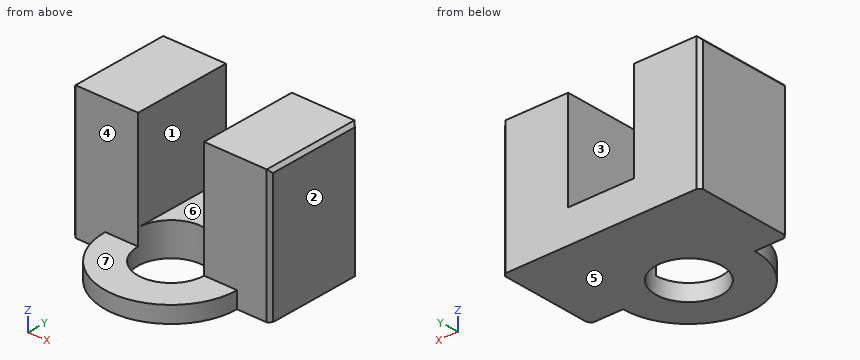
from build123d import *

# Parameters (mm, degrees)
BOSS_EXTRUDE1_DEPTH = 30
SKETCH2_R           = 20
BOSS_EXTRUDE2_DEPTH = 5
SKETCH3_R           = 10
CUT_EXTRUDE1_DEPTH  = 20
CHAMFER1_SIZE       = 1


with BuildPart() as part:
    # Sketch1 → Boss-Extrude1 (new body)
    with BuildSketch(Plane(origin=(0, 0, 0), x_dir=(1, 0, 0), z_dir=(0, 1, 0))):
        Polygon((-30, 0), (-30, -40), (-10, -40), (-10, -10), (10, -10), (10, -40), (30, -40), (30, 0), align=None)
    extrude(amount=BOSS_EXTRUDE1_DEPTH)

    # Sketch2 → Boss-Extrude2 (add)
    with BuildSketch(Plane.XY):
        Circle(SKETCH2_R)
    extrude(amount=BOSS_EXTRUDE2_DEPTH)

    # Sketch3 → Cut-Extrude1 (cut)
    with BuildSketch(Plane.XY):
        Circle(SKETCH3_R)
    extrude(amount=CUT_EXTRUDE1_DEPTH, mode=Mode.SUBTRACT)

    # Chamfer1
    chamfer1_edges = [part.edges().sort_by_distance(p)[0] for p in [
        (-30, 0, 20),
        (30, 15, 40),
        (-30, 15, 40),
        (30, 30, 20),
        (30, 0, 20),
        (-30, 30, 20),
    ]]
    chamfer(chamfer1_edges, length=CHAMFER1_SIZE)


solid = part.part
Here's how the part is built. I have some questions about the finished solid (model axes, mm). Face numbers are marked on the shaded views. A direction names the side the tool comes from. Round coordinates to 2 decimals unless told otherwise and drop trailing zeros. Order: outer loops, then holes, each group sorted by start corner. A loop starts at its lowest first (then second) coordinate and runs counter-clockwise, first axis right, second up. Notation, with made-up numbers: (84, 52.25) -> (110, 52.25) arc R19 cw to (110, 79.25) -> close; hole circle Ø11 at (-8.75, 84). An arc over 180 degrees is marked (long way). Use CSV: the item, a comma, the result in double quotes.
1. I want a section at D-D on y = 18. List the corners of the cut face in (x, z) for me.
Recorded:
outline,"(-30, 0) -> (30, 0) -> (30, 39) -> (29, 40) -> (10, 40) -> (10, 10) -> (-10, 10) -> (-10, 40) -> (-29, 40) -> (-30, 39) -> close"
2. Which directions (+Z, -Z, +X, -X, +Y, -Y) give clear straight access to the entire face, cutting with the end or side of a thin tool? Please do the marked faces 5, 6 and 7.
Recorded:
face 5,"-Z, +X, -X, +Y, -Y"
face 6,"+Z, +Y, -Y"
face 7,"+Z, +X, -X, -Y"
3. I want a section at A-A on y = 6. List the corners of the cut face in (x, z) for me, and give its area (3 significant figures).
Recorded:
outline,"(-30, 0) -> (-8, 0) -> (-8, 10) -> (-10, 10) -> (-10, 40) -> (-29, 40) -> (-30, 39) -> close; (8, 0) -> (30, 0) -> (30, 39) -> (29, 40) -> (10, 40) -> (10, 10) -> (8, 10) -> close"
area,"1,640 mm2"
4. I need wall thicknesses on line 1 along X through (y, z) = (28, 37.5); line 2 along Y through (x, z) = (0, 4); line 3 along Y through (x, z) = (0, 6.5). Which ranges of each line are inside material? Lowest first, please.
Recorded:
line 1,"x = -30 to -10, 10 to 30"
line 2,"y = -20 to -10, 10 to 30"
line 3,"y = 10 to 30"
5. I want a section at B-B on x = 0. List the corners of the cut face in (y, z) for me, and give its area (3 significant figures).
Recorded:
outline,"(-20, 0) -> (-10, 0) -> (-10, 5) -> (-20, 5) -> close; (10, 0) -> (30, 0) -> (30, 10) -> (10, 10) -> close"
area,"250 mm2"
6. I want a section at C-C on z = 34.5. List the corners of the cut face in (x, y) for me, and give its area (3 significant figures).
Recorded:
outline,"(-30, 1) -> (-29, 0) -> (-10, 0) -> (-10, 30) -> (-29, 30) -> (-30, 29) -> close; (10, 0) -> (29, 0) -> (30, 1) -> (30, 29) -> (29, 30) -> (10, 30) -> close"
area,"1,200 mm2"
7. I'm going to push flat-ended pins straight in: P1, Ø8, axis at x = -21, z = 4.5, coming from the -Y side; P2, Ø6, axis at x = -3.5, y = -11.5, coming from the +Z side; P3, Ø9.5, axis at x = -23, z = 11, coming from the -Y side. Where does each tip first touch, or does it pass through?
Recorded:
P1,"stops at y = -10.54"
P2,"stops at z = 5"
P3,"stops at y = 0"
8. Thinking about a two-plate mould opening in X: for the marked faces 1, 2, 3 and 4, which applies, pulls with the +X half, pulls with the -X half, needs draft (parallel to the pull), parting line crosses it, or undercut?
Recorded:
face 1,"undercut"
face 2,"pulls with the +X half"
face 3,"undercut"
face 4,"needs draft"
